CAD build for the part. Positions are in the model's coordinates, mm. Face numbers are marked on the shaded views. A direction names the side the tool comes from. Coordinates: 2 decimals unless noted, no trailing zeros. Loops run counter-clockwise (first coordinate to the right, second up) from the corner with the lowest first, then second, coordinate; pieces in that order, holes last.
1) Pin check, flat tips, straight feed: pin 1 Ø2 at (x, y) = (-3, -3) entering from -Z; pin 2 Ø2 at (y, z) = (-3, 26.5) entering from -X; pin 3 Ø1.5 at (x, z) = (1.5, 23) entering from +Y. Stop position of each tip, or through.
2) Saw through at C-C, the plane x = -2. Write the cut outline in (y, z), and give its area (3 significant figures).
3) Wall check: line 1 along Y through (x, z) = (0, 39.25) (3 decimals); line 2 along Z through (x, y) = (3.25, 2.5); line 3 along X through (y, z) = (-0.25, 42.5). Give the ranges that are in metal, low to high.
4) Saw through at B-B, the plane y = 3.25. Write the cut outline in (x, z), and give its area (3 significant figures).
5) Which spindle directions (+Z, -Z, +X, -X, +Y, -Y) get a long thin tool onto all of the face, cutting with end or side? Do the marked faces 1, 2 and 3. Say none if no direction does.
6) Saw through at A-A, the plane z = 43.5. Write the cut outline in (x, y) (3 decimals).
```python
from build123d import *

# Parameters (mm, degrees)
F0_R     = 4
F1_DEPTH = 6
F2_W     = 8
F2_H     = 8
F3_DEPTH = 15
F4_R     = 4
F5_DEPTH = 25
F6_R     = 1.575
F7_DEPTH = 10


with BuildPart() as f1:
    # F0 (on Top) → F1 (new body)
    with BuildSketch(Plane.XY):
        Circle(F0_R)
    extrude(amount=F1_DEPTH)

    # F2 (on face) → F3 (join)
    with BuildSketch(Plane.XY.offset(6)):
        Rectangle(F2_W, F2_H)
    extrude(amount=F3_DEPTH)

    # F4 (on face) → F5 (join)
    with BuildSketch(Plane.XY.offset(21)):
        Circle(F4_R)
    extrude(amount=F5_DEPTH)

    # F6 (on face) → F7 (cut)
    with BuildSketch(Plane.XY.offset(46)):
        Circle(F6_R)
    extrude(amount=-F7_DEPTH, mode=Mode.SUBTRACT)


solid = f1.part
```
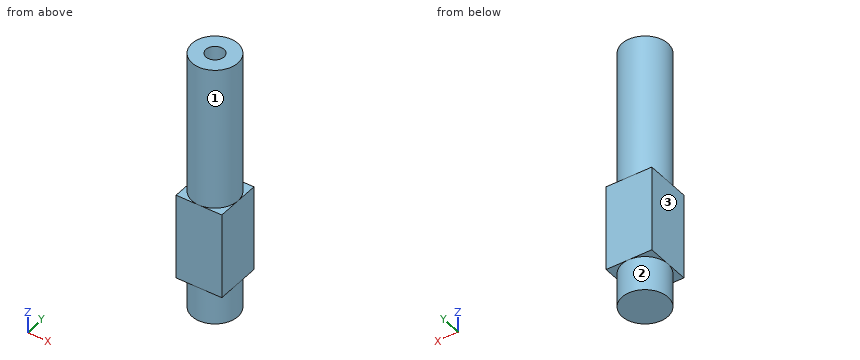
Data:
1. pin 1: stops at z = 0
1. pin 2: stops at x = -3.46
1. pin 3: stops at y = 3.93
2. outline: (-4, 6) - (-3.46, 6) - (-3.46, 0) - (3.46, 0) - (3.46, 6) - (4, 6) - (4, 21) - (3.46, 21) - (3.46, 46) - (-3.46, 46) - (-3.46, 21) - (-4, 21) - close
2. area: 335 mm2
3. line 1: y = -4 to -1.575, 1.575 to 4
3. line 2: z = 6 to 21
3. line 3: x = -3.99 to -1.56, 1.56 to 3.99
4. outline: (-4, 6) - (-2.33, 6) - (-2.33, 0) - (2.33, 0) - (2.33, 6) - (4, 6) - (4, 21) - (2.33, 21) - (2.33, 46) - (-2.33, 46) - (-2.33, 21) - (-4, 21) - close
4. area: 265 mm2
5. face 1: +Z
5. face 2: -Z
5. face 3: +Z, -Z, -X, +Y, -Y
6. outline: circle Ø8 at (0, 0); hole circle Ø3.15 at (0, 0)
